Part model, mm, in its own coordinate system. Face numbers are marked on the shaded views. A direction names the side the tool comes from. Round coordinates to 2 decimals unless told otherwise and drop trailing zeros. Loops run counter-clockwise (first coordinate to the right, second up) from the corner with the lowest first, then second, coordinate; pieces in that order, holes last. Notation, with made-up numbers: M 83.5,12.5 L 109.5,12.5 A24 ccw 109.5,22.5 Z; hole C 37,24 d7. An arc over 180 degrees is marked long. Put each result on its own line as item: value. Start each with the question number.
1) Drop a flat-ended pin along its axis: pin 1 Ø1.4 at (x, y) = (-1, -1) entering from +Z. Give the stop position or say it passes through.
2) Slice it at D-D on z = 1.75. Give the cut face in (x, y), then the cut area to 3 significant figures.
3) Which spindle directions (+Z, -Z, +X, -X, +Y, -Y) get a long thin tool onto all of the face, cutting with end or side? Do the marked faces 4 and 5. Say none if no direction does.
4) Slice it at C-C on z = 6. Give the cut face in (x, y).
5) Slice it at A-A on x = 0. Give the cut face in (y, z) (3 decimals), then the cut area to 3 significant figures.
6) Probe line 1 along Y through (x, z) = (0, 7.45) (3 decimals); line 2 along Z through (x, y) = (-0.5, 0.75); line 3 along Z through (x, y) = (2.75, 2.75). List the from-to ranges inside material, lowest first.
7) Pull direction X, two halves, no side cores. Call the marked faces 1, 2 and 3: +X half, -X half, draft (parallel to the pull), parting line (faces both ways), or undercut.
```python
from build123d import *

# Parameters (mm, degrees)
SKETCH1_R           = 4.91
BOSS_EXTRUDE1_DEPTH = 3
SKETCH4_R           = 3.75
BOSS_EXTRUDE3_DEPTH = 3.84
SKETCH2_R           = 3.75
SKETCH2_R_2         = 2.375
BOSS_EXTRUDE2_DEPTH = 1.76


with BuildPart() as part:
    # Sketch1 → Boss-Extrude1 (new body)
    with BuildSketch(Plane.XY):
        Circle(SKETCH1_R)
    extrude(amount=BOSS_EXTRUDE1_DEPTH)

    # Sketch4 → Boss-Extrude3 (add)
    with BuildSketch(Plane.XY.offset(3)):
        Circle(SKETCH4_R)
    extrude(amount=BOSS_EXTRUDE3_DEPTH)

    # Sketch2 → Boss-Extrude2 (add)
    with BuildSketch(Plane.XY.offset(6.84)):
        Circle(SKETCH2_R)
        Circle(SKETCH2_R_2, mode=Mode.SUBTRACT)
    extrude(amount=BOSS_EXTRUDE2_DEPTH)


solid = part.part
```
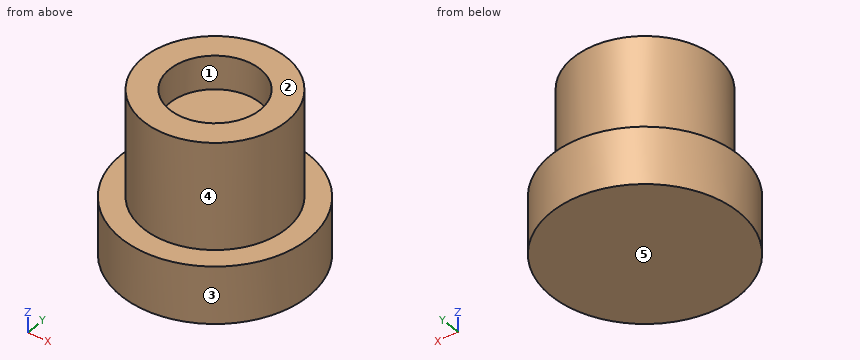
Recorded:
1. pin 1: stops at z = 6.84
2. outline: C 0,0 d9.82
2. area: 75.7 mm2
3. face 4: +Z
3. face 5: -Z, +X, -X, +Y, -Y
4. outline: C 0,0 d7.5
5. outline: M -4.91,0 L 4.91,0 L 4.91,3 L 3.75,3 L 3.75,8.6 L 2.375,8.6 L 2.375,6.84 L -2.375,6.84 L -2.375,8.6 L -3.75,8.6 L -3.75,3 L -4.91,3 Z
5. area: 63.1 mm2
6. line 1: y = -3.75 to -2.375, 2.375 to 3.75
6. line 2: z = 0 to 6.84
6. line 3: z = 0 to 3
7. face 1: undercut
7. face 2: draft
7. face 3: parting line
